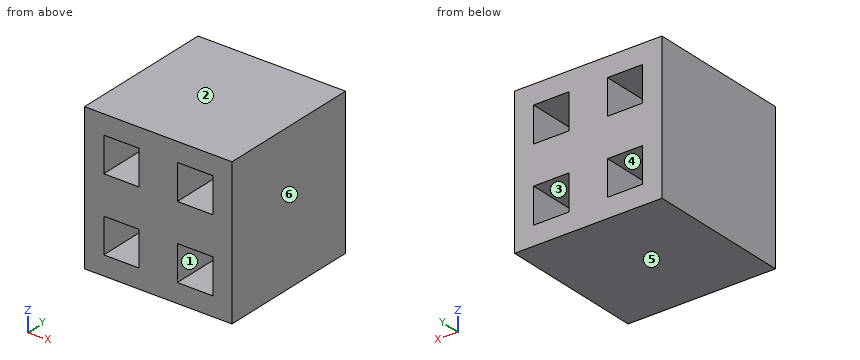
```python
from build123d import *

# Parameters (mm, degrees)
F1_DEPTH = 75.946


with BuildPart() as f1:
    # F0 (on Front) → F1 (new body, symmetric)
    with BuildSketch(Plane.XZ):
        Polygon((76.458305, 75.877115), (-76.458305, 75.877115), (-56.450146, 56.021046), (-20.00816, 56.021046), (-20.00816, 19.85607), (0, 0), (19.80776, 19.657193), (19.80776, 56.219922), (56.650545, 56.219922), align=None)
        Polygon((-56.450146, 56.021046), (-76.458305, 75.877115), (-76.458305, -75.877115), (-56.451009, -56.021903), (-56.451009, -19.855212), (-20.007296, -19.855212), (0, 0), (-20.00816, 19.85607), (-56.450146, 19.85607), align=None)
        Polygon((-56.451009, -56.021903), (-76.458305, -75.877115), (76.458305, -75.877115), (56.650545, -56.219922), (19.80776, -56.219922), (19.80776, -19.657193), (0, 0), (-20.007296, -19.855212), (-20.007296, -56.021903), align=None)
        Polygon((76.458305, -75.877115), (76.458305, 75.877115), (56.650545, 56.219922), (56.650545, 19.657193), (19.80776, 19.657193), (0, 0), (19.80776, -19.657193), (56.650545, -19.657193), (56.650545, -56.219922), align=None)
    extrude(amount=F1_DEPTH, both=True)


solid = f1.part
```
The listing builds one solid part. Answer for the finished solid, in the listing's coordinates (mm). Face numbers are marked on the shaded views. A direction names the side the tool comes from. Give positions to 0.01 mm unless a question says otherwise; leave off trailing zeros. Order: outer loops, then holes, each group sorted by start corner. A loop starts at its lowest first (then second) coordinate and runs counter-clockwise, first axis right, second up. Notation, with made-up numbers: (33, 37) - (39, 37) arc R35 cw to (39, 72) - close; hole circle Ø5 at (59, 33). An arc over 180 degrees is marked (long way). Use one line per item in the form item = value. Start each with the question number.
(1) A cutting plane is placed at A-A, the plane z = -40. Write down the section's boundary in (x, y).
(2) A cutting plane is placed at C-C, the plane y = -21. Write down the section's boundary in (x, z), then the cut area to 3 significant figures.
(3) The mould has two halves that part along Z. Classify the marked faces 3, 4, 5 and 6: released by +Z, released by -Z, zero draft, split by the parting line, or undercut.
(4) Consider line 1 (X direction, y = 63.5, z = 30); line 2 (Z direction, x = 37, y = 21); line 3 (Z direction, x = -36.5, y = -34.5). Determine where each line is inside the solid, lowest interval first. Write a range as from..to.
(5) For the marked faces 1 and 2, determine the directions among +Z, -Z, +X, -X, +Y, -Y from which every point of the face is accessible in a straight line to the end or side of a thin tool.
(6) A cutting plane is placed at B-B, the plane x = -45.5. Write down the section's boundary in (y, z).
Ans:
q1.outline = (-76.46, -75.95) - (-56.45, -75.95) - (-56.45, 75.95) - (-76.46, 75.95) - close; (-20.01, -75.95) - (19.81, -75.95) - (19.81, 75.95) - (-20.01, 75.95) - close; (56.65, -75.95) - (76.46, -75.95) - (76.46, 75.95) - (56.65, 75.95) - close
q2.outline = (-76.46, -75.88) - (76.46, -75.88) - (76.46, 75.88) - (-76.46, 75.88) - close; hole (-56.45, -56.02) - (-20.01, -56.02) - (-20.01, -19.86) - (-56.45, -19.86) - close; hole (-56.45, 19.86) - (-20.01, 19.86) - (-20.01, 56.02) - (-56.45, 56.02) - close; hole (19.81, -56.22) - (56.65, -56.22) - (56.65, -19.66) - (19.81, -19.66) - close; hole (19.81, 19.66) - (56.65, 19.66) - (56.65, 56.22) - (19.81, 56.22) - close
q2.area = 17,900 mm^2
q3.face_3 = undercut
q3.face_4 = undercut
q3.face_5 = released by -Z
q3.face_6 = zero draft
q4.line_1 = -76.46..-56.45, -20.01..19.81, 56.65..76.46
q4.line_2 = -75.88..-56.22, -19.66..19.66, 56.22..75.88
q4.line_3 = -75.88..-56.02, -19.86..19.86, 56.02..75.88
q5.face_1 = +Y, -Y
q5.face_2 = +Z, +X, -X, +Y, -Y
q6.outline = (-75.95, -75.88) - (75.95, -75.88) - (75.95, -56.02) - (-75.95, -56.02) - close; (-75.95, -19.86) - (75.95, -19.86) - (75.95, 19.86) - (-75.95, 19.86) - close; (-75.95, 56.02) - (75.95, 56.02) - (75.95, 75.88) - (-75.95, 75.88) - close
